CAD build for the part. Positions are in the model's coordinates, mm. Face numbers are marked on the shaded views. A direction names the side the tool comes from. Round coordinates to 2 decimals unless told otherwise and drop trailing zeros. Order: outer loops, then holes, each group sorted by start corner. A loop starts at its lowest first (then second) coordinate and runs counter-clockwise, first axis right, second up. Notation, with made-up numbers: (-18, 40.25) - (35, 40.25) arc R23 cw to (35, 49.25) - close; hole circle Ø5 at (-18, 38.25). An arc over 180 degrees is marked (long way). Write item = value, one per line.
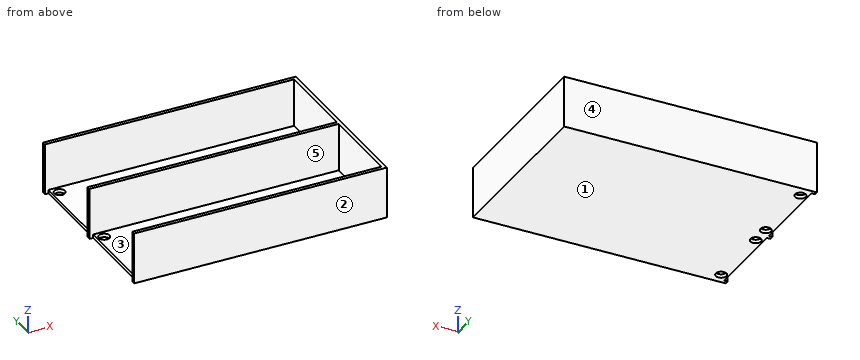
from build123d import *

# Parameters (mm, degrees)
SKETCH1_W           = 142
SKETCH1_H           = 100
BOSS_EXTRUDE1_DEPTH = 2
BOSS_EXTRUDE2_DEPTH = 27
SKETCH4_W           = 2
SKETCH4_H           = 47
CUT_EXTRUDE1_DEPTH  = 3
SKETCH5_R           = 3
CUT_EXTRUDE4_DEPTH  = 30


with BuildPart() as part:
    # Sketch1 → Boss-Extrude1 (new body)
    with BuildSketch(Plane.XY):
        with Locations((8.448668202, -3.21033452)):
            Rectangle(SKETCH1_W, SKETCH1_H)
    extrude(amount=BOSS_EXTRUDE1_DEPTH)

    # Sketch3 → Boss-Extrude2 (add)
    with BuildSketch(Plane.XY.offset(2)):
        Polygon((-62.551331798, -53.21033452), (79.448668202, -53.21033452), (79.448668202, 46.78966548), (-62.551331798, 46.78966548), (-62.551331798, 44.78966548), (77.448668202, 44.78966548), (77.448668202, -2.21033452), (-62.551331798, -2.21033452), (-62.551331798, -4.21033452), (77.448668202, -4.21033452), (77.448668202, -51.21033452), (-62.551331798, -51.21033452), align=None)
    extrude(amount=BOSS_EXTRUDE2_DEPTH)

    # Sketch4 → Cut-Extrude1 (cut, through all)
    with BuildSketch(Plane.XY.offset(2)):
        with Locations((-61.551331798, 21.28966548)):
            Rectangle(SKETCH4_W, SKETCH4_H)
        with Locations((-61.551331798, -27.71033452)):
            Rectangle(SKETCH4_W, SKETCH4_H)
    extrude(amount=-CUT_EXTRUDE1_DEPTH, mode=Mode.SUBTRACT)

    # Sketch5 → Cut-Extrude4 (cut, through all)
    with BuildSketch(Plane(origin=(0, 0, 0), x_dir=(-1, 0, 0), z_dir=(0, 0, -1))):
        with Locations((56.551331798, 40.28966548)):
            Circle(SKETCH5_R)
        with Locations((56.551331798, 2.28966548)):
            Circle(SKETCH5_R)
        with Locations((56.551331798, -8.71033452)):
            Circle(SKETCH5_R)
        with Locations((56.551331798, -46.71033452)):
            Circle(SKETCH5_R)
    extrude(amount=-CUT_EXTRUDE4_DEPTH, mode=Mode.SUBTRACT)


solid = part.part
(1) Band-saw the part on A-A on x = -42.5. List the corners of the cut face in (y, z), plus the area to 3 significant figures.
Solved:
outline = (-53.21, 0) - (46.79, 0) - (46.79, 29) - (44.79, 29) - (44.79, 2) - (-2.21, 2) - (-2.21, 29) - (-4.21, 29) - (-4.21, 2) - (-51.21, 2) - (-51.21, 29) - (-53.21, 29) - close
area = 362 mm²
(2) Probe line 1 along Y through (x, z) = (59.5, 27.25); line 2 along Z through (x, y) = (30.5, -48.5); line 3 along X through (y, z) = (-32, 5). List the from-to ranges inside material, lowest first.
Solved:
line_1 = -53.21 to -51.21, -4.21 to -2.21, 44.79 to 46.79
line_2 = 0 to 2
line_3 = 77.45 to 79.45
(3) Drop flat-ended pins along their axis: pin 1 (3.5 mm diameter, centred on x = -56.55, y = 40.29, fed in from -Z); pin 2 (14 mm diameter, centred on x = -16.5, y = 26, fed in from +Z); pin 3 (2 mm diameter, centred on y = -15.5, z = 19.5, fed in from -X); pin 4 (0.6 mm diameter, centred on y = 24, z = 0.5, fed in from -X). Give the stop position or say it passes through.
Solved:
pin_1 = through
pin_2 = 2
pin_3 = 77.45
pin_4 = -60.55
(4) Band-saw the part on B-B on z = 9. List the corners of the cut face in (x, y), plus the area to 3 significant figures.
Solved:
outline = (-62.55, -53.21) - (79.45, -53.21) - (79.45, 46.79) - (-62.55, 46.79) - (-62.55, 44.79) - (77.45, 44.79) - (77.45, -2.21) - (-62.55, -2.21) - (-62.55, -4.21) - (77.45, -4.21) - (77.45, -51.21) - (-62.55, -51.21) - close
area = 1,040 mm²
(5) Pull direction Y, two halves, no side cores. Call the marked faces 1, 2 and 3: released by +Y, released by -Y, zero draft, split by the parting line, or undercut.
Solved:
face_1 = zero draft
face_2 = released by -Y
face_3 = undercut
(6) Band-saw the part on C-C on y = -27. List the corners of the cut face in (x, z).
Solved:
outline = (-60.55, 0) - (79.45, 0) - (79.45, 29) - (77.45, 29) - (77.45, 2) - (-60.55, 2) - close
(7) Tool access for the marked faces 4 and 5: list every direction of +Z, -Z, +X, -X, +Y, -Y with a clear straight run to the whole face (end or side of a thin tool).
Solved:
face_4 = +Z, -Z, +X, -X, +Y
face_5 = +Z, -X
